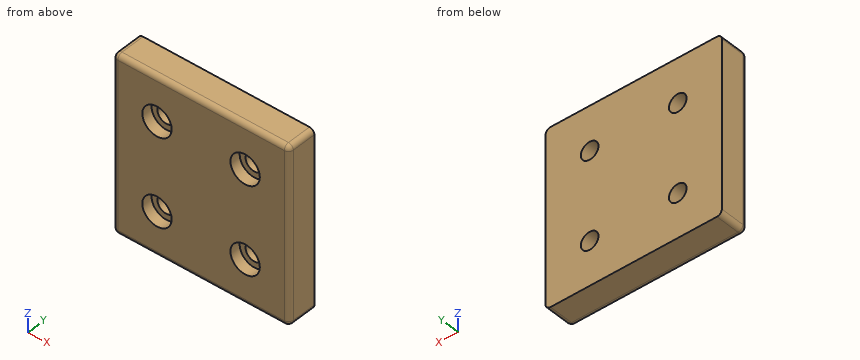
Solid Edge part; units mm, degrees
sketch "Sketch1" plane through (0, 0, 0) normal (0, -1, 0) x (1, 0, 0)
  line L0 (45, 45) -> (-45, 45)
  line L1 (-45, 45) -> (-45, -45)
  line L2 (-45, -45) -> (45, -45)
  line L3 (45, -45) -> (45, 45)
  dimension "D1" = 45
extrude "Protrusion1" add sketch "Sketch1" against normal blind 15
fillet "Redondeo_1" radius 2.5 8 edges at (45, 0, 0) (0, 0, 45) (-45, 0, 0) (0, 0, -45) (45, 7.5, 45) (45, 7.5, -45) (-45, 7.5, -45) (-45, 7.5, 45)
hole "Agujero_1" at (-22.5, 0, 22.5) direction (0, 1, 0) diameter 9 end up to next counterbore diameter 15 counterbore depth 5.5
pattern_linear "Pattern1" count 2 spacing 45 along (1, 0, 0) count 2 spacing 45 along (0, 0, -1) of "Agujero_1"
properties part number "1983-1100-C03"
Source: CAD feature listing. Evaluate the final solid. Frame: model axes, mm. Coordinates: 2 decimals unless noted, no trailing zeros. Loops run counter-clockwise (first coordinate to the right, second up) from the corner with the lowest first, then second, coordinate; pieces in that order, holes last. Notation, with made-up numbers: (37, -29.75) - (92, -29.75) arc R13 ccw to (92, -19.75) - close; hole circle Ø2 at (-31.5, -27). An arc over 180 degrees is marked (long way). Return JSON: item names as keys, results as strings.
Q1. Section B-B, the plane y = 10.25. Return loops of the section in (x, z), plus the area to 3 significant figures.
Results:
{"outline": "(-45, -42.5) arc R2.5 ccw to (-42.5, -45) - (42.5, -45) arc R2.5 ccw to (45, -42.5) - (45, 42.5) arc R2.5 ccw to (42.5, 45) - (-42.5, 45) arc R2.5 ccw to (-45, 42.5) - close; hole circle Ø9 at (-22.5, -22.5); hole circle Ø9 at (-22.5, 22.5); hole circle Ø9 at (22.5, -22.5); hole circle Ø9 at (22.5, 22.5)", "area": "7,840 mm2"}
Q2. Section C-C, the plane x = -22.5. Return loops of the section in (y, z), plus the area to 3 significant figures.
Results:
{"outline": "(0, -42.5) arc R2.5 ccw to (2.5, -45) - (15, -45) - (15, -27) - (5.5, -27) - (5.5, -30) - (0, -30) - close; (0, -15) - (5.5, -15) - (5.5, -18) - (15, -18) - (15, 18) - (5.5, 18) - (5.5, 15) - (0, 15) - close; (0, 30) - (5.5, 30) - (5.5, 27) - (15, 27) - (15, 45) - (2.5, 45) arc R2.5 ccw to (0, 42.5) - close", "area": "1,010 mm2"}
Q3. Contact query for flat-ended pins moving along their axis: P1, Ø4.5, axis at x = 22.5, z = -22, coming from the -Y side; P2, Ø12, axis at x = -22.5, z = 22.5, coming from the -Y side. Output: stop coordinate, or through.
Results:
{"P1": "through", "P2": "y = 5.5"}
Q4. Section A-A, the plane z = -22.5. Return loops of the section in (x, y), plus the area to 3 significant figures.
Results:
{"outline": "(-45, 2.5) arc R2.5 ccw to (-42.5, 0) - (-30, 0) - (-30, 5.5) - (-27, 5.5) - (-27, 15) - (-45, 15) - close; (-18, 5.5) - (-15, 5.5) - (-15, 0) - (15, 0) - (15, 5.5) - (18, 5.5) - (18, 15) - (-18, 15) - close; (27, 5.5) - (30, 5.5) - (30, 0) - (42.5, 0) arc R2.5 ccw to (45, 2.5) - (45, 15) - (27, 15) - close", "area": "1,010 mm2"}
Q5. Section D-D, the plane y = 3.75. Return loops of the section in (x, z).
Results:
{"outline": "(-45, -42.5) arc R2.5 ccw to (-42.5, -45) - (42.5, -45) arc R2.5 ccw to (45, -42.5) - (45, 42.5) arc R2.5 ccw to (42.5, 45) - (-42.5, 45) arc R2.5 ccw to (-45, 42.5) - close; hole circle Ø15 at (-22.5, -22.5); hole circle Ø15 at (-22.5, 22.5); hole circle Ø15 at (22.5, -22.5); hole circle Ø15 at (22.5, 22.5)"}
Q6. Material intervals for line 1 along Z through (x, y) = (-22.5, 9); line 2 along X through (y, z) = (3.4, 22.5), sorted ascending.
Results:
{"line 1": "-45 to -27, -18 to 18, 27 to 45", "line 2": "-45 to -30, -15 to 15, 30 to 45"}
